The model under review builds one solid part; all positions refer to its coordinate system, in mm. Coordinates: 2 decimals unless noted, no trailing zeros. Order: outer loops, then holes, each group sorted by start corner. A loop starts at its lowest first (then second) coordinate and runs counter-clockwise, first axis right, second up.
```python
from build123d import *

# Parameters (mm, degrees)
SKETCH1_W                        = 876.3
SKETCH1_H                        = 222.25
BOSS_EXTRUDE1_DEPTH              = 6.35
F_10_CLEARANCE_HOLE1_D           = 5.6134
F_10_CLEARANCE_HOLE1_CSINK_D     = 6.8834
F_10_CLEARANCE_HOLE1_CSINK_ANGLE = 90
CUT_EXTRUDE1_DEPTH               = 492.335738065


with BuildPart() as part:
    # Sketch1 → Boss-Extrude1 (new body)
    with BuildSketch(Plane.XY):
        with Locations((0, 111.125)):
            Rectangle(SKETCH1_W, SKETCH1_H)
    extrude(amount=BOSS_EXTRUDE1_DEPTH)

    # #10 Clearance Hole1 (through all)
    with Locations(Plane.XY.offset(6.35)):
        with Locations((-50.8, 19.05), (50.8, 19.05)):
            CounterSinkHole(F_10_CLEARANCE_HOLE1_D / 2, F_10_CLEARANCE_HOLE1_CSINK_D / 2, counter_sink_angle=F_10_CLEARANCE_HOLE1_CSINK_ANGLE)

    # Sketch5 → Cut-Extrude1 (cut, through all)
    with BuildSketch(Plane.XY.offset(6.35)):
        with BuildLine():
            Line((112.7125, 234.95), (315.9125, 234.95))
            Line((315.9125, 234.95), (315.9125, 222.25))
            ThreePointArc((315.9125, 222.25), (298.814601737, 218.957245657), (284.1625, 209.55))
            ThreePointArc((284.1625, 209.55), (269.510398263, 200.142754343), (252.4125, 196.85))
            Line((252.4125, 196.85), (176.2125, 196.85))
            ThreePointArc((176.2125, 196.85), (159.114601737, 200.142754343), (144.4625, 209.55))
            ThreePointArc((144.4625, 209.55), (129.810398263, 218.957245657), (112.7125, 222.25))
            Line((112.7125, 222.25), (112.7125, 234.95))
        make_face()
    cut_extrude1 = extrude(amount=-CUT_EXTRUDE1_DEPTH, mode=Mode.SUBTRACT)

    # Mirror1: Cut-Extrude1 across plane
    add(cut_extrude1.mirror(Plane(origin=(0, 0, 0), x_dir=(0, 0, 1), z_dir=(1, 0, 0))), mode=Mode.SUBTRACT)


solid = part.part
```
(1) Wall thickness on probe 1 along X at (y, z) = (19.05, 1.95); probe 2 along Y at (x, z) = (50.8, 1.25); probe 3 along X at (y, z) = (206.5, 2.25): over which ranges is each line inside the solid? List them lowest first.
A:
probe 1: x = -438.15 to -53.61, -47.99 to 47.99, 53.61 to 438.15
probe 2: y = 0 to 16.24, 21.86 to 222.25
probe 3: x = -438.15 to -280.62, -148.01 to 148.01, 280.62 to 438.15
(2) For pin 1 Ø3 at (x, z) = (-210, 4.5) entering from +Y, flat-tipped, find the tip position at first contact; note if it passes through.
A:
pin 1: stops at y = 196.85
(3) We need section A-A, the plane z = 4.75. Count the separate pieces of the cut face and the enclosed holes in it, and give its area (3 significant figures).
A:
separate pieces: 1
enclosed holes: 2
area: 188,000 mm2
(4) We need section B-B, the plane x = 195. Write out the cut boundary in (y, z).
A:
outline: (0, 0) - (196.85, 0) - (196.85, 6.35) - (0, 6.35) - close
